Source: CAD feature listing. Evaluate the final solid. Frame: model axes, mm. Face numbers are marked on the shaded views. Coordinates: 2 decimals unless noted, no trailing zeros. Write each loop counter-clockwise with the first axis right and the second up, starting at its lowest first coordinate (ties: lowest second). Pieces come first, ordered by that corner, then holes. Notation, with made-up numbers: M -20,46.25 L -1,46.25 A24 ccw -1,62.25 Z; hole C -17.5,61 d2. An arc over 180 degrees is marked long. Answer as CSV lines item,"result". Start each with the question number.
1. Section C-C on y = 1.25. Count the separate pieces of the cut face and the enclosed holes in it, plus the area to 3 significant figures.
2. Line query: probe 1 along Z at (x, y) = (-21.5, 0.3); probe 2 along Z at (x, y) = (-22.25, 3.15); probe 3 along Z at (x, y) = (-28.25, 1.65). Output: solid intervals per line, ascending. Write a range as [from, to].
3. Section D-D on x = -30. Return the cut outline in (y, z).
4. Contact query for a flat-ended pin moving along its axis: pin 1 Ø1 at (x, y) = (-19, 4.5) entering from +Z. Output: stop coordinate, or through.
5. Mould query, pull axis X, two halves, no side actions, for the marked faces 1, 2 and 3. Classes: pulls with the +X half, pulls with the -X half, needs draft (parallel to the pull), parting line crosses it, or undercut.
6. Section A-A on x = -25.5. Return the cut outline in (y, z).
7. Section B-B on z = -21.75. Return the cut outline in (x, y), plus the area to 3 significant figures.
Autodesk Inventor part; units mm, degrees
ref_plane "YZ Plane" through (0, 0, 0) normal (1, 0, 0) x (0, 1, 0)
ref_plane "XZ Plane" through (0, 0, 0) normal (0, 1, 0) x (-1, 0, 0)
ref_plane "XY Plane" through (0, 0, 0) normal (0, 0, 1) x (1, 0, 0)
sketch "스케치1" plane through (0, 0, 0) normal (0, 1, 0) x (-1, 0, 0)
  circle A0 centre (13.7314, -40.8752) radius 1.55
  circle A1 centre (29.2877, -40.8752) radius 1.55
  circle A2 centre (29.2877, -25.3189) radius 1.55
  circle A3 centre (13.7314, -25.3189) radius 1.55
  circle A4 centre (21.5095, -33.0971) radius 13.9
  circle A5 centre (21.5095, -22.0971) radius 1.55
  circle A6 centre (32.5095, -33.0971) radius 1.55
  circle A7 centre (21.5095, -44.0971) radius 1.55
  circle A8 centre (10.5095, -33.0971) radius 1.55
  circle A9 centre (21.5095, -33.0971) radius 5.2
  circle A10 centre (29.2877, -40.8752) radius 1.35
  circle A11 centre (21.5095, -44.0971) radius 1.35
  circle A12 centre (13.7314, -40.8752) radius 1.35
  circle A13 centre (10.5095, -33.0971) radius 1.35
  circle A14 centre (13.7314, -25.3189) radius 1.35
  circle A15 centre (21.5095, -22.0971) radius 1.35
  circle A16 centre (29.2877, -25.3189) radius 1.35
  circle A17 centre (32.5095, -33.0971) radius 1.35
  point P0 (0, 0)
  point P1 (21.5095, -33.0971)
  dimension "d3" = 2.7
  dimension "d4" = 2.7
  dimension "d5" = 2.7
  dimension "d6" = 2.7
  dimension "d7" = 2.7
  dimension "d8" = 2.7
  dimension "d9" = 2.7
  dimension "d10" = 2.7
extrude "돌출1" add sketch "스케치1" along normal blind 6 contours A0 | A1 | A2 | A3 | A4 | A5 | A6 | A7 | A8
properties part number "long_horn1" material "PMMA 플라스틱"
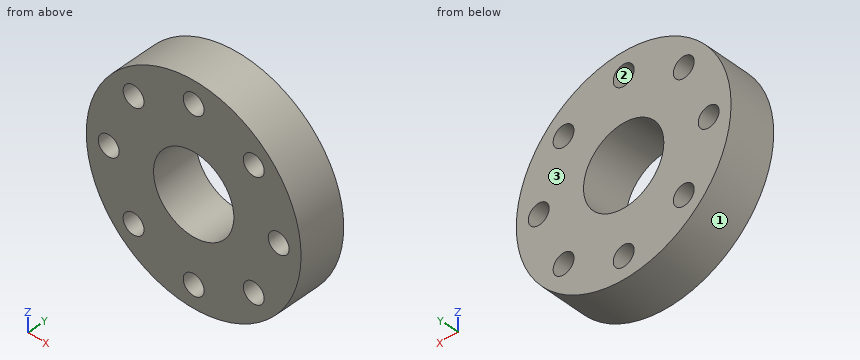
Values:
1,separate pieces,"1"
1,enclosed holes,"9"
1,area,"476 mm²"
2,probe 1,"[-47, -45.45], [-42.75, -38.3], [-27.9, -23.45], [-20.75, -19.2]"
2,probe 2,"[-46.98, -45.23], [-42.97, -38.24], [-27.95, -23.23], [-20.97, -19.22]"
2,probe 3,"[-45.25, -41.74], [-40.01, -26.18], [-24.46, -20.94]"
3,outline,"M 0,-44.1 L 6,-44.1 L 6,-42.02 L 0,-42.02 Z; M 0,-39.73 L 6,-39.73 L 6,-26.47 L 0,-26.47 Z; M 0,-24.17 L 6,-24.17 L 6,-22.09 L 0,-22.09 Z"
4,pin 1,"z = -19.34"
5,face 1,"parting line crosses it"
5,face 2,"undercut"
5,face 3,"needs draft"
6,outline,"M 0,-46.41 L 6,-46.41 L 6,-36.43 L 0,-36.43 Z; M 0,-29.76 L 6,-29.76 L 6,-19.78 L 0,-19.78 Z"
7,outline,"M -29.54,0 L -22.81,0 L -22.81,6 L -29.54,6 Z; M -20.2,0 L -13.48,0 L -13.48,6 L -20.2,6 Z"
7,area,"80.7 mm²"
